For this review, take the finished solid that the model builds, in its own axes (mm). Face numbers are marked on the shaded views. A direction names the side the tool comes from. Give positions to 0.01 mm unless a question says otherwise; leave off trailing zeros. Write each loop counter-clockwise with the first axis right and the second up, starting at its lowest first coordinate (ties: lowest second). Pieces come first, ordered by that corner, then holes.
1) We need section B-B on y = 128. Give the boundary of the cut face in (x, z), and give its area (3 significant figures).
2) Wall thickness on line 1 along Y through (x, z) = (9.5, 32) (3 decimals); line 2 along X through (y, z) = (133.5, 60.9); line 3 along Y through (x, z) = (3.25, 63) (3 decimals): over which ranges is each line inside the solid? List them lowest first.
3) We need section D-D on z = 9.5. Give the boundary of the cut face in (x, y) (3 decimals), and give its area (3 significant figures).
4) Draft analysis for pull direction Z (two halves, no side actions). For the marked faces 3 and 4, state which applies: pulls with the +Z half, pulls with the -Z half, needs draft (parallel to the pull), parting line crosses it, or undercut.
5) Machinability: for the marked faces 1 and 2, which of the approach directions +Z, -Z, +X, -X, +Y, -Y give a long, thin tool a straight path to every point of the face, cutting with its end or side? Answer none if there is none.
6) For P1, Ø3, axis at x = -1, y = 140, coming from the -Z side; P2, Ø1.6, axis at y = 5.5, z = 56, coming from the +X side; P3, Ø12, axis at y = 64, z = 35.5, coming from the -X side, all flat-tipped, find the tip position at first contact; note any pin that passes through.
7) We need section C-C on x = -11. Give the boundary of the cut face in (y, z) (3 decimals), and give its area (3 significant figures).
8) We need section A-A on z = 60.9. Give the boundary of the cut face in (x, y) (3 decimals).
from build123d import *
from build123d.topology import SkipClean

# Parameters (mm, degrees)
SKETCH4_R           = 2
BOSS_EXTRUDE1_DEPTH = 140
SKETCH5_W           = 29.5
SKETCH5_H           = 13.79
BOSS_EXTRUDE3_DEPTH = 79.9
SKETCH6_W           = 75.9
SKETCH6_H           = 9.7
CUT_EXTRUDE1_DEPTH  = 27.5
SKETCH7_W           = 23.5
SKETCH7_H           = 26
CUT_EXTRUDE2_DEPTH  = 3
SKETCH8_R           = 2
BOSS_EXTRUDE4_DEPTH = 22.95
SKETCH12_R          = 8.5
BOSS_EXTRUDE6_DEPTH = 15.01
SKETCH13_R          = 8.5
BOSS_EXTRUDE7_DEPTH = 4
SKETCH14_R          = 6.5
CUT_EXTRUDE3_DEPTH  = 12


with BuildPart() as part:
    # Sketch4 → Boss-Extrude1 (new body)
    with BuildSketch(Plane(origin=(0, 0, 0), x_dir=(1, 0, 0), z_dir=(0, 1, 0))):
        with Locations(Location((0, -39.95, 0), (0, 0, 270))):
            Circle(SKETCH4_R)
    extrude(amount=BOSS_EXTRUDE1_DEPTH)

    # Sketch5 → Boss-Extrude3 (add)
    with BuildSketch(Plane.XY):
        Rectangle(SKETCH5_W, SKETCH5_H)
    extrude(amount=BOSS_EXTRUDE3_DEPTH)

    # Sketch6 → Cut-Extrude1 (cut)
    with BuildSketch(Plane(origin=(14.75, 0, 0), x_dir=(0, 0, -1), z_dir=(1, 0, 0))):
        with Locations((-39.95, 0)):
            Rectangle(SKETCH6_W, SKETCH6_H)
    extrude(amount=-CUT_EXTRUDE1_DEPTH, mode=Mode.SUBTRACT)

    # Sketch7 → Cut-Extrude2 (cut)
    with BuildSketch(Plane(origin=(0, 6.895, 0), x_dir=(1, 0, 0), z_dir=(0, 1, 0))):
        with Locations((3, -60.9)):
            Rectangle(SKETCH7_W, SKETCH7_H)
    extrude(amount=-CUT_EXTRUDE2_DEPTH, mode=Mode.SUBTRACT)

    # Sketch8 → Boss-Extrude4 (add)
    with SkipClean():  # the faces are left unmerged after this step: merging them gives an invalid solid
        with BuildSketch(Plane.XY.offset(37.95)):
            with Locations((0, 140)):
                Circle(SKETCH8_R)
        extrude(amount=BOSS_EXTRUDE4_DEPTH)

    # Sketch12 → Boss-Extrude6 (add)
    with SkipClean():  # the faces are left unmerged after this step: merging them gives an invalid solid
        with BuildSketch(Plane(origin=(0, 140, 0), x_dir=(1, 0, 0), z_dir=(0, 1, 0))):
            with Locations(Location((0, -60.9, 0), (0, 0, 270))):
                Circle(SKETCH12_R)
        extrude(amount=-BOSS_EXTRUDE6_DEPTH)

    # Sketch13 → Boss-Extrude7 (add)
    with SkipClean():  # the faces are left unmerged after this step: merging them gives an invalid solid
        with BuildSketch(Plane(origin=(0, 140, 0), x_dir=(1, 0, 0), z_dir=(0, 1, 0))):
            with Locations(Location((0, -60.9, 0), (0, 0, 270))):
                Circle(SKETCH13_R)
        extrude(amount=BOSS_EXTRUDE7_DEPTH)

    # Sketch14 → Cut-Extrude3 (cut)
    with SkipClean():  # the faces are left unmerged after this step: merging them gives an invalid solid
        with BuildSketch(Plane.XZ.offset(-124.99)):
            with Locations(Location((0, 60.9, 0), (0, 0, 270))):
                Circle(SKETCH14_R)
        extrude(amount=-CUT_EXTRUDE3_DEPTH, mode=Mode.SUBTRACT)


solid = part.part
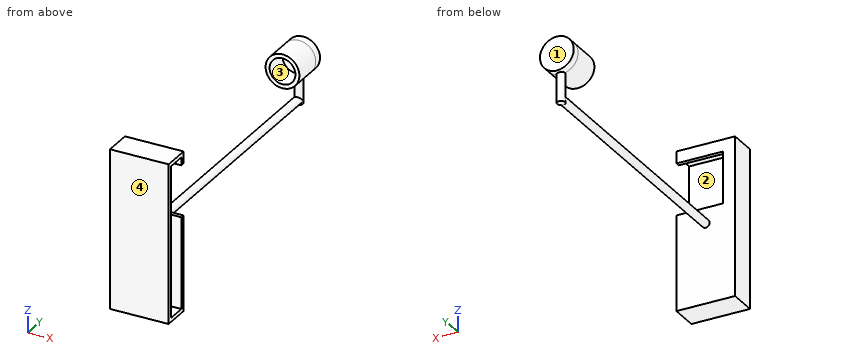
Results list:
1. outline: circle Ø17 at (0, 60.9); circle Ø4 at (0, 39.95); hole circle Ø13 at (0, 60.9)
1. area: 107 mm2
2. line 1: y = -6.895 to -4.85, 4.85 to 6.895
2. line 2: x = -8.5 to -6.5, 6.5 to 8.5
2. line 3: y = -6.895 to -4.85, 136.99 to 144
3. outline: (-14.75, -6.895) - (14.75, -6.895) - (14.75, -4.85) - (-12.75, -4.85) - (-12.75, 4.85) - (14.75, 4.85) - (14.75, 6.895) - (-14.75, 6.895) - close
3. area: 140 mm2
4. face 3: undercut
4. face 4: needs draft
5. face 1: +Z, -Z, +X, -X, +Y
5. face 2: +X
6. P1: stops at z = 37.95
6. P2: stops at x = -8.75
6. P3: stops at x = -2
7. outline: (-6.895, 0) - (6.895, 0) - (6.895, 79.9) - (-6.895, 79.9) - close; hole (-4.85, 2) - (4.85, 2) - (4.85, 77.9) - (-4.85, 77.9) - close
7. area: 366 mm2
8. outline: (-14.75, -6.895) - (14.75, -6.895) - (14.75, -4.85) - (-12.75, -4.85) - (-12.75, 4.85) - (-8.75, 4.85) - (-8.75, 6.895) - (-14.75, 6.895) - close; (-8.5, 124.99) - (-6.5, 124.99) - (-6.5, 136.99) - (6.5, 136.99) - (6.5, 124.99) - (8.5, 124.99) - (8.5, 144) - (-8.5, 144) - close
